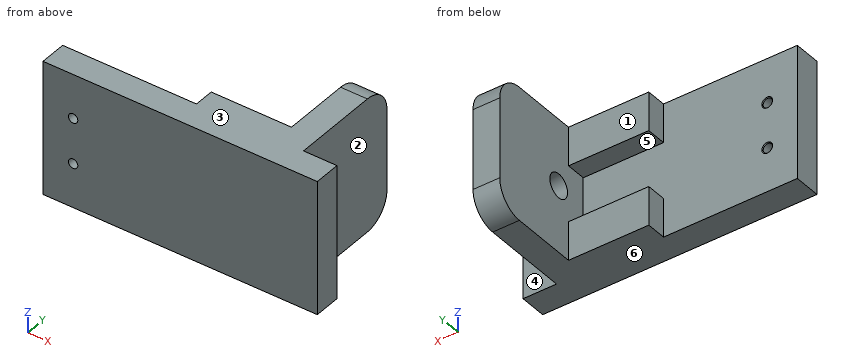
from build123d import *

# Parameters (mm, degrees)
SCHIZZO1_W                          = 205
SCHIZZO1_H                          = 100
ESTRUSIONE_ESTRUSIONE1_DEPTH        = 20
ESTRUSIONE_ESTRUSIONE2_START        = 20
ESTRUSIONE_ESTRUSIONE2_DEPTH        = 85
TAGLIO_ESTRUSIONE1_DEPTH            = 156.020159979
TAGLIO_ESTRUSIONE1_DEPTH_BACK       = 156.020159979
SCHIZZO4_W                          = 60
SCHIZZO4_H                          = 70
TAGLIO_ESTRUSIONE2_START            = 77.5
SCHIZZO6_R                          = 9
TAGLIO_ESTRUSIONE2_DEPTH            = 80
FORO_FILETTATO_M8X1_0_1_D           = 7
FORO_FILETTATO_M8X1_0_1_CSINK_D     = 8.05
FORO_FILETTATO_M8X1_0_1_CSINK_ANGLE = 82


with BuildPart() as part:
    # Schizzo1 → Estrusione-Estrusione1 (new body)
    with BuildSketch(Plane(origin=(0, 0, 0), x_dir=(1, 0, 0), z_dir=(0, 1, 0))):
        Rectangle(SCHIZZO1_W, SCHIZZO1_H)
    extrude(amount=ESTRUSIONE_ESTRUSIONE1_DEPTH)

    # Schizzo2 → Estrusione-Estrusione2 (add)
    with BuildSketch(Plane(origin=(0, 0, 0), x_dir=(1, 0, 0), z_dir=(0, 1, 0)).offset(ESTRUSIONE_ESTRUSIONE2_START)):
        Polygon((77.5, 50), (77.5, -50), (-2.5, -50), (-2.5, -21), (57.5, -21), (57.5, 21), (-2.5, 21), (-2.5, 50), align=None)
    extrude(amount=ESTRUSIONE_ESTRUSIONE2_DEPTH)

    # Schizzo4 → Taglio-Estrusione1 (cut, two sides: drawn at the far end of the back side and taken through both)
    with BuildSketch(Plane.XY.offset(-TAGLIO_ESTRUSIONE1_DEPTH_BACK)):
        with Locations((27.5, 70)):
            Rectangle(SCHIZZO4_W, SCHIZZO4_H)
    extrude(amount=TAGLIO_ESTRUSIONE1_DEPTH + TAGLIO_ESTRUSIONE1_DEPTH_BACK, mode=Mode.SUBTRACT)

    # Schizzo6 → Taglio-Estrusione2 (cut)
    with BuildSketch(Plane(origin=(0, 0, 0), x_dir=(0, 0, -1), z_dir=(1, 0, 0)).offset(TAGLIO_ESTRUSIONE2_START)):
        with Locations((0, 45)):
            Circle(SCHIZZO6_R)
        with BuildLine():
            Line((-50, 85), (-50, 105))
            Line((-50, 105), (-30, 105))
            ThreePointArc((-30, 105), (-44.142135624, 99.142135624), (-50, 85))
        make_face()
        with BuildLine():
            Line((30, 105), (50, 105))
            Line((50, 105), (50, 85))
            ThreePointArc((50, 85), (44.142135624, 99.142135624), (30, 105))
        make_face()
    extrude(amount=-TAGLIO_ESTRUSIONE2_DEPTH, mode=Mode.SUBTRACT)

    # Foro filettato M8x1.0-1 (through all)
    with Locations(Plane(origin=(0, 20, 0), x_dir=(1, 0, 0), z_dir=(0, 1, 0))):
        with Locations((-80, -17), (-80, 17)):
            CounterSinkHole(FORO_FILETTATO_M8X1_0_1_D / 2, FORO_FILETTATO_M8X1_0_1_CSINK_D / 2, counter_sink_angle=FORO_FILETTATO_M8X1_0_1_CSINK_ANGLE)


solid = part.part
Build history of the part. All positions in model axes, mm. Face numbers are marked on the shaded views. A direction names the side the tool comes from. Round coordinates to 2 decimals unless told otherwise and drop trailing zeros. Loops run counter-clockwise (first coordinate to the right, second up) from the corner with the lowest first, then second, coordinate; pieces in that order, holes last. Notation, with made-up numbers: (-1.5, -16.5) -> (47.5, -16.5) arc R19 ccw to (47.5, 11.5) -> close; hole circle Ø4 at (1.25, -2). An arc over 180 degrees is marked (long way). Answer in a Markdown table with one row per item.
Item 1: Which spindle directions (+Z, -Z, +X, -X, +Y, -Y) get a long thin tool onto all of the face, cutting with end or side? Do the marked faces 1, 2 and 3. Say none if no direction does.
Answers below:
| item | result |
|---|---|
| face 1 | +Z, -Z, -X, +Y |
| face 2 | +Z, -Z, +X, +Y |
| face 3 | +Z, +X, -X, +Y, -Y |
Item 2: Pin check, flat tips, straight feed: pin 1 (12 mm diameter, centred on y = 28, z = 38.5, fed in from -X); pin 2 (11 mm diameter, centred on x = -80, z = 17, fed in from +Y); pin 3 (20.5 mm diameter, centred on y = 45, z = 0, fed in from -X). Stop position of each tip, or through.
Answers below:
| item | result |
|---|---|
| pin 1 | stops at x = -2.5 |
| pin 2 | stops at y = 20 |
| pin 3 | stops at x = 57.5 |
Item 3: Drill centre lines: L1, parallel to Z at x = -80, y = 12; L2, parallel to Y at x = 70, z = 0; L3, parallel to X at y = 8, z = 17. Where is each one in solid material? Low to high. Write a range as [from, to].
Answers below:
| item | result |
|---|---|
| L1 | z = [-50, -20.5], [-13.5, 13.5], [20.5, 50] |
| L2 | y = [0, 36], [54, 105] |
| L3 | x = [-102.5, -83.5], [-76.5, 102.5] |
Item 4: Saw through at C-C (z = 26.5). Write the cut outline in (x, y).
Answers below:
| item | result |
|---|---|
| outline | (-102.5, 0) -> (102.5, 0) -> (102.5, 20) -> (77.5, 20) -> (77.5, 105) -> (57.5, 105) -> (57.5, 35) -> (-2.5, 35) -> (-2.5, 20) -> (-102.5, 20) -> close |
Item 5: Saw through at A-A (z = -17). Write the cut outline in (x, y) (3 decimals).
Answers below:
| item | result |
|---|---|
| outline | (-102.5, 0) -> (-83.5, 0) -> (-83.5, 19.396) -> (-84.025, 20) -> (-102.5, 20) -> close; (-76.5, 0) -> (102.5, 0) -> (102.5, 20) -> (77.5, 20) -> (77.5, 105) -> (57.5, 105) -> (57.5, 20) -> (-75.975, 20) -> (-76.5, 19.396) -> close |
Item 6: Mould opens along Z. For the marked faces 4, 5 and 6 say: +Z half, -Z half, draft (parallel to the pull), parting line (faces both ways), or undercut.
Answers below:
| item | result |
|---|---|
| face 4 | draft |
| face 5 | undercut |
| face 6 | -Z half |
Item 7: Saw through at B-B (x = -80). Write the cut outline in (y, z) (3 decimals).
Answers below:
| item | result |
|---|---|
| outline | (0, -50) -> (20, -50) -> (20, -21.025) -> (19.396, -20.5) -> (0, -20.5) -> close; (0, -13.5) -> (19.396, -13.5) -> (20, -12.975) -> (20, 12.975) -> (19.396, 13.5) -> (0, 13.5) -> close; (0, 20.5) -> (19.396, 20.5) -> (20, 21.025) -> (20, 50) -> (0, 50) -> close |
Item 8: Saw through at D-D (y = 41.5). Write the cut outline in (x, z).
Answers below:
| item | result |
|---|---|
| outline | (57.5, -50) -> (77.5, -50) -> (77.5, -8.29) -> (57.5, -8.29) -> close; (57.5, 8.29) -> (77.5, 8.29) -> (77.5, 50) -> (57.5, 50) -> close |
